Geometry: final body of the model. Coordinates: model frame, mm. Face numbers are marked on the shaded views. Give positions to 0.01 mm unless a question says otherwise; leave off trailing zeros. Write each loop counter-clockwise with the first axis right and the second up, starting at its lowest first coordinate (ties: lowest second). Pieces come first, ordered by that corner, then holes.
Q1. Mould query, pull axis Y, two halves, no side actions, for the marked faces 1, 2 and 3. Classes: +Y half, -Y half, draft (parallel to the pull), parting line (faces both ways), or undercut.
Q2. Section A-A (x = 762). Return the cut outline in (y, z), plus the area to 3 significant figures.
Q3. Section D-D (z = 266). Return the cut outline in (x, y), plus the area to 3 significant figures.
Q4. Section B-B (y = 0). Return the cut outline in (x, z).
Q5. Section C-C (x = -762). Return the cut outline in (y, z).
Q6. Pin query (flat end, axial travel): pin 1 Ø5 at (x, y) = (287.5, -325.5) entering from -Z. Return the tip coordinate at first contact, or that it passes through.
Q7. Line query: line 1 (Y direction, x = 762, z = 389); line 2 (Z direction, x = -67, y = -273.5); line 3 (X direction, y = -46, z = 824). Output: solid intervals per line, ascending.
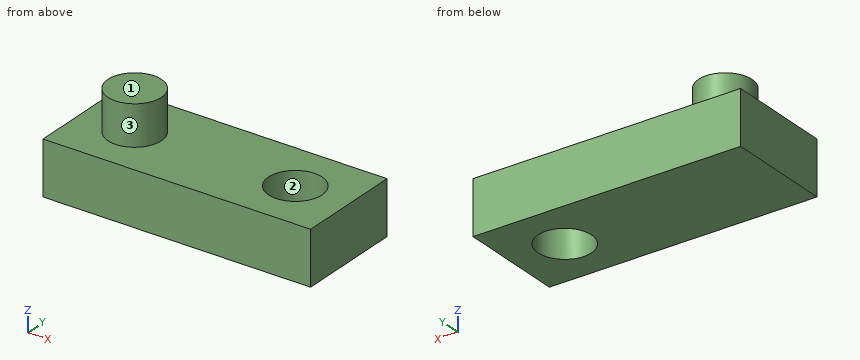
from build123d import *

# Parameters (mm, degrees)
SKETCH1_W           = 2540
SKETCH1_H           = 1016
BOSS_EXTRUDE1_DEPTH = 508
SKETCH2_R           = 254
BOSS_EXTRUDE2_DEPTH = 381
SKETCH3_R           = 254
CUT_EXTRUDE2_DEPTH  = 508


with BuildPart() as part:
    # Sketch1 → Boss-Extrude1 (new body)
    with BuildSketch(Plane.XY):
        Rectangle(SKETCH1_W, SKETCH1_H)
    extrude(amount=BOSS_EXTRUDE1_DEPTH)

    # Sketch2 → Boss-Extrude2 (add)
    with BuildSketch(Plane.XY.offset(508)):
        with Locations((-762, 0)):
            Circle(SKETCH2_R)
    extrude(amount=BOSS_EXTRUDE2_DEPTH)

    # Sketch3 → Cut-Extrude2 (cut)
    with BuildSketch(Plane.XY.offset(508)):
        with Locations((762, 0)):
            Circle(SKETCH3_R)
    extrude(amount=-CUT_EXTRUDE2_DEPTH, mode=Mode.SUBTRACT)


solid = part.part
Computed:
1. face 1: draft
1. face 2: undercut
1. face 3: parting line
2. outline: (-508, 0) - (-254, 0) - (-254, 508) - (-508, 508) - close; (254, 0) - (508, 0) - (508, 508) - (254, 508) - close
2. area: 258,000 mm2
3. outline: (-1270, -508) - (1270, -508) - (1270, 508) - (-1270, 508) - close; hole circle Ø508 at (762, 0)
3. area: 2,380,000 mm2
4. outline: (-1270, 0) - (508, 0) - (508, 508) - (-508, 508) - (-508, 889) - (-1016, 889) - (-1016, 508) - (-1270, 508) - close; (1016, 0) - (1270, 0) - (1270, 508) - (1016, 508) - close
5. outline: (-508, 0) - (508, 0) - (508, 508) - (254, 508) - (254, 889) - (-254, 889) - (-254, 508) - (-508, 508) - close
6. pin 1: stops at z = 0
7. line 1: y = -508 to -254, 254 to 508
7. line 2: z = 0 to 508
7. line 3: x = -1011.8 to -512.2
